Check sheet for the modelled part. Datum: model origin and axes. Units: mm. A direction names the side the tool comes from. Round coordinates to 2 decimals unless told otherwise and drop trailing zeros. Write each loop counter-clockwise with the first axis right and the second up, starting at its lowest first coordinate (ties: lowest second). Pieces come first, ordered by that corner, then holes. Notation, with made-up numbers: (21, 49.5) -> (36, 49.5) arc R12 cw to (36, 61.5) -> close; hole circle Ø3 at (-26, 86.25). An arc over 180 degrees is marked (long way). One line per item, written item: value.
from build123d import *

# Parameters (mm, degrees)
CROQUIS1_W                 = 5
CROQUIS1_H                 = 5
SALIENTE_EXTRUIR1_DEPTH    = 50
CROQUIS2_R                 = 1.5
SALIENTE_EXTRUIR2_DEPTH    = 5
CORTAR_EXTRUIR1_DEPTH      = 56.167925464
CORTAR_EXTRUIR1_DEPTH_BACK = 56.167925464
CROQUIS3_W                 = 3
CROQUIS3_H                 = 8


with BuildPart() as part:
    # Croquis1 → Saliente-Extruir1 (new body)
    with BuildSketch(Plane(origin=(0, 0, 0), x_dir=(1, 0, 0), z_dir=(0, 1, 0))):
        with Locations((0, -0.104885861)):
            Rectangle(CROQUIS1_W, CROQUIS1_H)
    extrude(amount=-SALIENTE_EXTRUIR1_DEPTH)

    # Croquis2 → Saliente-Extruir2 (add, symmetric)
    with BuildSketch(Plane(origin=(0, 0, 0), x_dir=(0, 0, -1), z_dir=(1, 0, 0))):
        with BuildLine():
            Line((10.5, -3.5), (-10.5, -3.5))
            ThreePointArc((-10.5, -3.5), (-11.914213562, -2.914213562), (-12.5, -1.5))
            Line((-12.5, -1.5), (-12.5, 1.5))
            ThreePointArc((-12.5, 1.5), (-11.914213562, 2.914213562), (-10.5, 3.5))
            Line((-10.5, 3.5), (10.5, 3.5))
            ThreePointArc((10.5, 3.5), (11.914213562, 2.914213562), (12.5, 1.5))
            Line((12.5, 1.5), (12.5, -1.5))
            ThreePointArc((12.5, -1.5), (11.914213562, -2.914213562), (10.5, -3.5))
        make_face()
        with Locations((-8.5, 0)):
            Circle(CROQUIS2_R, mode=Mode.SUBTRACT)
        with Locations((8.5, 0)):
            Circle(CROQUIS2_R, mode=Mode.SUBTRACT)
    extrude(amount=SALIENTE_EXTRUIR2_DEPTH, both=True)

    # Croquis3 → Cortar-Extruir1 (cut, two sides: drawn at the far end of the back side and taken through both)
    with BuildSketch(Plane(origin=(0, 3.5, 0), x_dir=(1, 0, 0), z_dir=(0, 1, 0)).offset(-CORTAR_EXTRUIR1_DEPTH_BACK)):
        with Locations((0, 8.5)):
            Rectangle(CROQUIS3_W, CROQUIS3_H)
        with Locations((0, -8.5)):
            Rectangle(CROQUIS3_W, CROQUIS3_H)
    extrude(amount=CORTAR_EXTRUIR1_DEPTH + CORTAR_EXTRUIR1_DEPTH_BACK, mode=Mode.SUBTRACT)


solid = part.part
Item 1: Sectioned sample at D-D (z = -5.75). Enter the section's corners in (x, y), then the cut area to 3 significant figures.
Result set:
outline: (-5, -3.5) -> (-1.5, -3.5) -> (-1.5, 3.5) -> (-5, 3.5) -> close; (1.5, -3.5) -> (5, -3.5) -> (5, 3.5) -> (1.5, 3.5) -> close
area: 49.0 mm^2
Item 2: Sectioned sample at C-C (x = -4.25). Enter the section's corners in (y, z).
Result set:
outline: (-3.5, -10.5) arc R2 ccw to (-1.5, -12.5) -> (1.5, -12.5) arc R2 ccw to (3.5, -10.5) -> (3.5, 10.5) arc R2 ccw to (1.5, 12.5) -> (-1.5, 12.5) arc R2 ccw to (-3.5, 10.5) -> close; hole circle Ø3 at (0, -8.5); hole circle Ø3 at (0, 8.5)
Item 3: Release check for a two-part mould opening along Y. For faces 1 (the flat face through (0, 3.5, 0)), 2 (the flat face through (-3, 0, -12.5)), 3 (the cylindrical face through (-3.3, -0.9, -7.3)) record: pulls with the +Y half, pulls with the -Y half, needs draft (parallel to the pull), parting line crosses it, or undercut.
Result set:
face 1: pulls with the +Y half
face 2: needs draft
face 3: undercut
Item 4: Tool access check on faces 4 (the flat face through (-1.5, -2, 9)), 5 (the flat face through (-2.5, -26, 0)), 6 (the cylindrical face through (3.27, 2.93, -11.9)), 7 (the flat face through (2.5, -26, 0)), 8 (the flat face through (0, -26, 2.605)). Record the directions out of +Z, -Z, +X, -X, +Y, -Y that give a thin tool (end or side, any length) a straight path to the whole face; none if there is none.
Result set:
face 4: +Z, +Y, -Y
face 5: +Z, -Z, -X, -Y
face 6: -Z, +X, -X, +Y
face 7: +Z, -Z, +X, -Y
face 8: +Z, +X, -X, -Y
Item 5: Sectioned sample at B-B (y = 0). Enter the section's corners in (x, z), then the cut area to 3 significant figures.
Result set:
outline: (-5, -12.5) -> (-1.5, -12.5) -> (-1.5, -10) -> (-5, -10) -> close; (-5, -7) -> (-1.5, -7) -> (-1.5, -4.5) -> (1.5, -4.5) -> (1.5, -7) -> (5, -7) -> (5, 7) -> (1.5, 7) -> (1.5, 4.5) -> (-1.5, 4.5) -> (-1.5, 7) -> (-5, 7) -> close; (-5, 10) -> (-1.5, 10) -> (-1.5, 12.5) -> (-5, 12.5) -> close; (1.5, -12.5) -> (5, -12.5) -> (5, -10) -> (1.5, -10) -> close; (1.5, 10) -> (5, 10) -> (5, 12.5) -> (1.5, 12.5) -> close
area: 160 mm^2
Item 6: Material ranges on line 1 along Z through (x, y) = (4.05, 0); line 2 along Y through (x, z) = (4.05, -8.5); line 3 along X through (y, z) = (-3, -8.5), recorded low to high.
Result set:
line 1: -12.5 to -10, -7 to 7, 10 to 12.5
line 2: -3.5 to -1.5, 1.5 to 3.5
line 3: -5 to -1.5, 1.5 to 5
Item 7: Sectioned sample at A-A (z = 8.5). Enter the section's corners in (x, y), then the cut area to 3 significant figures.
Result set:
outline: (-5, -3.5) -> (-1.5, -3.5) -> (-1.5, -1.5) -> (-5, -1.5) -> close; (-5, 1.5) -> (-1.5, 1.5) -> (-1.5, 3.5) -> (-5, 3.5) -> close; (1.5, -3.5) -> (5, -3.5) -> (5, -1.5) -> (1.5, -1.5) -> close; (1.5, 1.5) -> (5, 1.5) -> (5, 3.5) -> (1.5, 3.5) -> close
area: 28.0 mm^2
Item 8: Depth check by flat-ended pin: pin 1 (5.5 mm diameter, centred on y = -20, z = 0.5, fed in from -X); pin 2 (2 mm diameter, centred on x = 0, y = -31.5, fed in from +Z); pin 3 (1.5 mm diameter, centred on x = -0.5, y = -24.5, fed in from -Z). Enter the tip coordinate at first touch or a pass-through.
Result set:
pin 1: x = -2.5
pin 2: z = 2.6
pin 3: z = -2.4
